from build123d import *

# Parameters (mm, degrees)
SZKIC1_R                    = 3
DODANIE_WYCI_GNI_CIE2_DEPTH = 2.4
SZKIC2_R                    = 1.5
DODANIE_WYCI_GNI_CIE3_DEPTH = 10
ZAOKR_GLENIE2_R             = 1.2
WYTNIJ_WYCI_GNI_CIE1_DEPTH  = 1.94


with BuildPart() as part:
    # Szkic1 → Dodanie-wyciągnięcie2 (new body)
    with BuildSketch(Plane.XY):
        with Locations((-1.860516246, 2.732142857)):
            Circle(SZKIC1_R)
    extrude(amount=DODANIE_WYCI_GNI_CIE2_DEPTH)

    # Szkic2 → Dodanie-wyciągnięcie3 (add)
    with BuildSketch(Plane(origin=(0, 0, 0), x_dir=(-1, 0, 0), z_dir=(0, 0, -1))):
        with Locations((1.860516246, 2.732142857)):
            Circle(SZKIC2_R)
    extrude(amount=DODANIE_WYCI_GNI_CIE3_DEPTH)

    # Zaokrąglenie2
    zaokr_glenie2_edges = [part.edges().sort_by_distance(p)[0] for p in [
        (-4.860516246, 2.732142857, 2.4),
    ]]
    fillet(zaokr_glenie2_edges, radius=ZAOKR_GLENIE2_R)

    # Szkic3 → Wytnij-wyciągnięcie1 (cut)
    with BuildSketch(Plane.XY.offset(2.4)):
        with BuildLine():
            Line((-1.859548318, 2.959091853), (-0.575649693, 5.316481314))
            ThreePointArc((-0.575649693, 5.316481314), (-0.297886623, 5.158637444), (-0.039271083, 4.97106076))
            Line((-0.039271083, 4.97106076), (-1.329373025, 2.669425378))
            Line((-1.329373025, 2.669425378), (-0.183967515, 2.043621837))
            ThreePointArc((-0.183967515, 2.043621837), (-0.320475658, 1.776553075), (-0.499159616, 1.535654258))
            Line((-0.499159616, 1.535654258), (-1.621312108, 2.148584891))
            Line((-1.621312108, 2.148584891), (-2.819933608, 0.01015725))
            ThreePointArc((-2.819933608, 0.01015725), (-3.083174674, 0.117799023), (-3.33454353, 0.250826496))
            Line((-3.33454353, 0.250826496), (-2.145142944, 2.434706401))
            Line((-2.145142944, 2.434706401), (-3.258687897, 3.042935511))
            ThreePointArc((-3.258687897, 3.042935511), (-3.162842423, 3.328316127), (-3.009463836, 3.587359481))
            Line((-3.009463836, 3.587359481), (-1.859548318, 2.959091853))
        make_face()
    extrude(amount=-WYTNIJ_WYCI_GNI_CIE1_DEPTH, mode=Mode.SUBTRACT)


solid = part.part
Verification items for the finished model (mm, model axes). A direction names the side the tool comes from. Coordinates: 2 decimals unless noted, no trailing zeros. Order: outer loops, then holes, each group sorted by start corner. A loop starts at its lowest first (then second) coordinate and runs counter-clockwise, first axis right, second up. Notation, with made-up numbers: M 66.5,59 L 82.5,59 A26 cw 82.5,83 Z; hole C 80,52 d10. An arc over 180 degrees is marked long. Return JSON: item names as keys, results as strings.
1) Gauge pin test, flat ends, axial feed: pin 1 (2 mm diameter, centred on y = 2.5, z = -8, fed in from +X); pin 2 (3 mm diameter, centred on y = 5, z = -2, fed in from +X); pin 3 (3 mm diameter, centred on x = -4, z = -6, fed in from -Y). Record the tip position at first contact, or that the pin passes through.
Answer list:
{"pin 1": "x = -0.36", "pin 2": "x = -0.57", "pin 3": "y = 1.38"}
2) Cross-section at A-A, the plane z = -1.5. Record the boundary of the cut face in (x, y), and give its area (3 significant figures).
Answer list:
{"outline": "C -1.86,2.73 d3", "area": "7.07 mm2"}
3) Release check for a two-part mould opening along X. For faces 4 (the flat face through (-2.7, 3.6, 2.4)), 5 (the flat face through (-0.675, 3.836, 1.444)), 6 (the cylindrical face through (1, 3.63, 0.59)), 7 (the flat face through (-2.212, 1.094, 1.444)) record: +X half, -X half, draft (parallel to the pull), parting line (faces both ways), or undercut.
Answer list:
{"face 4": "draft", "face 5": "undercut", "face 6": "parting line", "face 7": "undercut"}
4) Access from +Z, -Z, +X, -X, +Y, -Y to the whole of each face (thin tool, end or side, straight path). Record for faces 1 (the flat face through (-2.694, 2.735, 1.444)), 2 (the flat face through (-3, 4, 0)), 3 (the flat face through (-2, 3, -10)).
Answer list:
{"face 1": "+Z", "face 2": "-Z", "face 3": "-Z, +X, -X, +Y, -Y"}
5) Thickness scan on L1, parallel to X at y = 3.75, z = 1.75; L2, parallel to Z at x = 0, y = 2.5; L3, parallel to Y at x = -2, z = -9.25. Record the ranges inside material, lowest first. Write a range as [from, to].
Answer list:
{"L1": "[-4.54, -1.43], [-0.72, 0.82]", "L2": "[0, 2.4]", "L3": "[1.24, 4.23]"}
